Here's how the part is built. I have some questions about the finished solid (model axes, mm). A direction names the side the tool comes from. Round coordinates to 2 decimals unless told otherwise and drop trailing zeros. Write each loop counter-clockwise with the first axis right and the second up, starting at its lowest first coordinate (ties: lowest second). Pieces come first, ordered by that corner, then holes. Notation, with made-up numbers: (82.5, 75.25) - (114.5, 75.25) arc R25 cw to (114.5, 106.25) - close; hole circle Ø5 at (-35.5, 81.5). An arc over 180 degrees is marked (long way). Write item = value, one per line. Start each with the question number.
Item 1: If we section it at A-A (x = 11.5): Please give me the cut outline in (y, z).
Item 2: If I drill on line 1 along Y through (x, z) = (48, 4); line 2 along Z through (x, y) = (-6, 1); line 3 along Y through (x, z) = (24, 48.5), over which ranges is the centre line in solid material (lowest first)? Write a range as [from, to].
Item 3: Thinking about a two-plate mould opening in Y: for faces 1 (the face through (24, 0, 92)), 2 (the face through (24, 15, 5)), 3 (the face through (45.802, 0.097, 4.93)), which applies, pulls with the +Y half, pulls with the -Y half, needs draft (parallel to the pull), parting line crosses it, or undercut?
Item 4: If we section it at C-C (z = 23): Please give me the cut outline in (x, y) (3 decimals).
Item 5: Which directions (+Z, -Z, +X, -X, +Y, -Y) give clear straight access to the entire face, cutting with the end or side of a thin tool? Please do faces 4 (the face through (17.08, 0.3, 21.9)), 5 (the face through (24, -15, 5)).
Item 6: For P1, Ø2, axis at x = 16, z = 13.5, coming from the +Y side; P2, Ø3, axis at x = 31.5, y = 9.5, coming from the +Z side; P3, Ø5, axis at x = 21, z = 75, coming from the -Y side; P4, Ø10, axis at y = 6, z = 67, coming from the +X side, each with a flat end and sliding along its axis, tell me the tip position at first contact or that it passes through.
Item 7: If we section it at B-B (z = 82): Please give me the cut outline in (x, y), and give its area (3 significant figures).
```python
from build123d import *

# Parameters (mm, degrees)
SKETCH1_R           = 2.2
BOSS_EXTRUDE1_DEPTH = 10
SKETCH2_R           = 6.925
BOSS_EXTRUDE2_DEPTH = 24
SKETCH3_R           = 5.95
BOSS_EXTRUDE3_DEPTH = 58
FILLET1_R           = 2
FILLET2_R           = 2
FILLET3_R           = 1
FILLET4_R           = 1


with BuildPart() as part:
    # Sketch1 → Boss-Extrude1 (new body)
    with BuildSketch(Plane.XY):
        with BuildLine():
            Line((0, 15), (48, 15))
            ThreePointArc((48, 15), (63, 0), (48, -15))
            Line((48, -15), (0, -15))
            ThreePointArc((0, -15), (-15, 0), (0, 15))
        make_face()
        Circle(SKETCH1_R, mode=Mode.SUBTRACT)
        with Locations((48, 0)):
            Circle(SKETCH1_R, mode=Mode.SUBTRACT)
    extrude(amount=BOSS_EXTRUDE1_DEPTH)

    # Sketch2 → Boss-Extrude2 (add)
    with BuildSketch(Plane.XY.offset(10)):
        with Locations((24, 0)):
            Circle(SKETCH2_R)
    extrude(amount=BOSS_EXTRUDE2_DEPTH)

    # Sketch3 → Boss-Extrude3 (add)
    with BuildSketch(Plane.XY.offset(34)):
        with Locations(Location((24, 0, 0), (0, 0, 180))):
            Circle(SKETCH3_R)
    extrude(amount=BOSS_EXTRUDE3_DEPTH)

    # Fillet1
    # the kernel refuses this fillet: 2 mm, written as the material it adds along each edge
    with BuildSketch(Plane(origin=(24, 0, 34), x_dir=(-1, 0, 0), z_dir=(0, 1, 0))) as fillet1_piece_1:
        with BuildLine():
            CenterArc((7.95, 1.71737445), FILLET1_R, 180, 59.169502568)
            Line((5.95, 1.71737445), (5.91, 1.71737445))
            Line((5.91, 1.71737445), (5.91, 0))
            Line((5.91, 0), (5.95, -0.04))
            ThreePointArc((5.95, -0.04), (6.4375, -0.04), (6.9045, -0.034347489))
            Line((6.9045, -0.034347489), (6.925, 0))
        make_face()
    revolve(axis=Axis((24, 0, 34), (0, 0, 1)))

    # Fillet2
    fillet2_edges = [part.edges().sort_by_distance(p)[0] for p in [
        (24, -6.925, 34),
    ]]
    fillet(fillet2_edges, radius=FILLET2_R)

    # Fillet3
    fillet3_edges = [part.edges().sort_by_distance(p)[0] for p in [
        (17.075, 0, 10),
    ]]
    fillet(fillet3_edges, radius=FILLET3_R)

    # Fillet4
    fillet4_edges = [part.edges().sort_by_distance(p)[0] for p in [
        (24, 15, 0),
        (63, 0, 0),
        (24, -15, 0),
        (-15, 0, 0),
    ]]
    fillet(fillet4_edges, radius=FILLET4_R)


solid = part.part
```
Reply:
q1.outline = (-15, 1) arc R1 ccw to (-14, 0) - (14, 0) arc R1 ccw to (15, 1) - (15, 10) - (-15, 10) - close
q2.line_1 = [-15, -2.2], [2.2, 15]
q2.line_2 = [0, 10]
q2.line_3 = [-5.95, 5.95]
q3.face_1 = needs draft
q3.face_2 = pulls with the +Y half
q3.face_3 = undercut
q4.outline = circle Ø13.85 at (24, 0)
q5.face_4 = +Z
q5.face_5 = +Z, -Z, +X, -X, -Y
q6.P1 = through
q6.P2 = 10
q6.P3 = -5.93
q6.P4 = 29.87
q7.outline = circle Ø11.9 at (24, 0)
q7.area = 111 mm2
